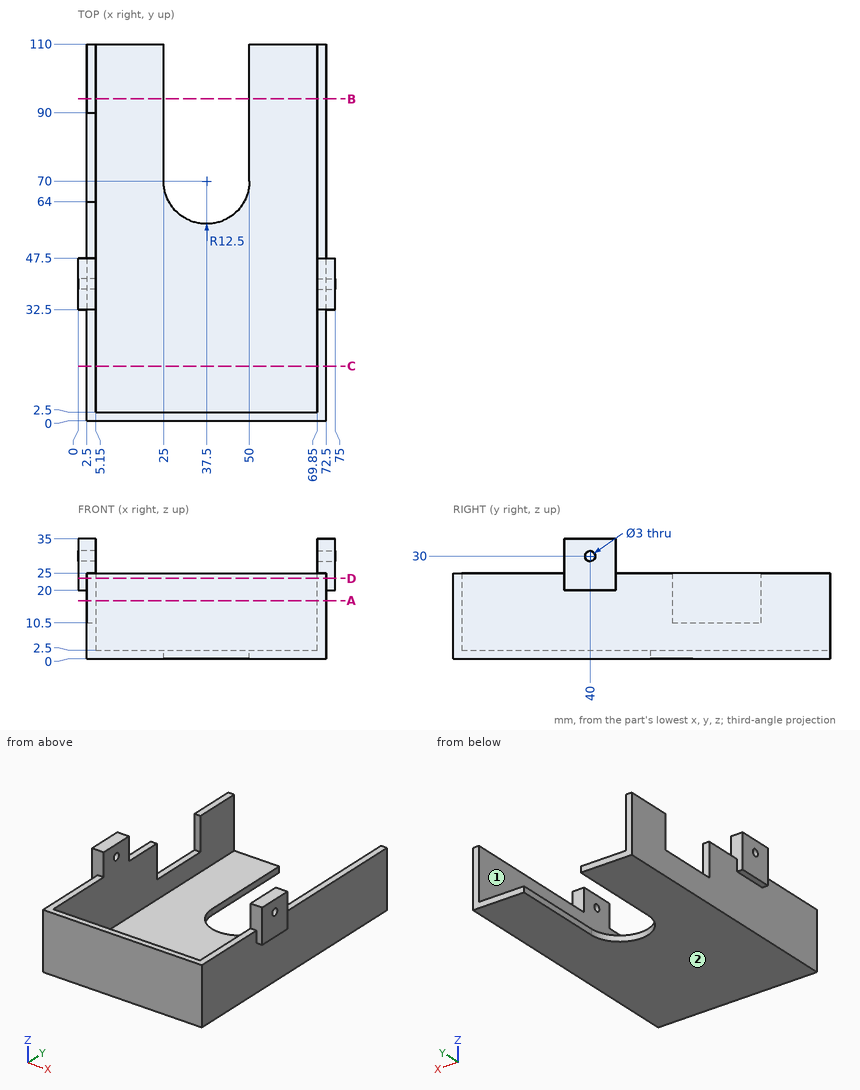
Geometry check sheet. Reference: drawing and pictorial views, mm from the part's lowest x, y, z. A direction names the side the tool comes from. Round coordinates to 2 decimals unless told otherwise and drop trailing zeros. Order: outer loops, then holes, each group sorted by start corner. A loop starts at its lowest first (then second) coordinate and runs counter-clockwise, first axis right, second up. Notation, with made-up numbers: (-26, -10) - (8, -10) arc R35 cw to (8, 23) - close; hole circle Ø10 at (26, 48.5). An arc over 180 degrees is marked (long way). Use a Markdown table: item, result. Add a question column.
1) Gauge pin test, flat ends, axial feed: P1, Ø1.3, axis at x = 3.5, y = 102, coming from the +Z side; P2, Ø0.8, axis at x = 4.5, y = 76.5, coming from the +Z side; P3, Ø5, axis at y = 40, z = 30, coming from the -X side; P4, Ø11, axis at x = 48, z = 14, coming from the +Y side. Record the tip position at first contact, or that the pin passes through.
2) Section check B-B (y = 94). Record the cut outline in (x, z).
3) Thickness scan on line 1 along X through (y, z) = (90, 7); line 2 along Y through (x, z) = (71.3, 30); line 3 along Z through (x, y) = (2.25, 40). Record the ranges inside material, lowest first.
4) Set-up check for the marked faces 1 and 2: record each of +Z, -Z, +X, -X, +Y, -Y from which the full face is reachable in a straight line by a thin tool's end or side.
5) Section check D-D (z = 23.5). Record the cut outline in (x, y).
6) Section check A-A (z = 17). Record the cut outline in (x, y), then the cut area to 3 significant figures.
7) Section check C-C (y = 16). Record the cut outline in (x, z).
Established:
| question | item | result |
|---|---|---|
| 1 | P1 | z = 25 |
| 1 | P2 | z = 10.5 |
| 1 | P3 | x = 0 |
| 1 | P4 | y = 2.5 |
| 2 | outline | (2.5, 0) - (25, 0) - (25, 2.5) - (5.15, 2.5) - (5.15, 25) - (2.5, 25) - close; (50, 0) - (72.5, 0) - (72.5, 25) - (69.85, 25) - (69.85, 2.5) - (50, 2.5) - close |
| 3 | line 1 | 2.5 to 5.15, 69.85 to 72.5 |
| 3 | line 2 | 32.5 to 38.5, 41.5 to 47.5 |
| 3 | line 3 | 20 to 28.5, 31.5 to 35 |
| 4 | face 1 | +Z, +Y |
| 4 | face 2 | -Z, +X, -X, +Y, -Y |
| 5 | outline | (0, 32.5) - (2.5, 32.5) - (2.5, 0) - (72.5, 0) - (72.5, 32.5) - (75, 32.5) - (75, 47.5) - (72.5, 47.5) - (72.5, 110) - (69.85, 110) - (69.85, 2.5) - (5.15, 2.5) - (5.15, 64) - (2.5, 64) - (2.5, 47.5) - (0, 47.5) - close; (2.5, 90) - (5.15, 90) - (5.15, 110) - (2.5, 110) - close |
| 6 | outline | (2.5, 0) - (72.5, 0) - (72.5, 110) - (69.85, 110) - (69.85, 2.5) - (5.15, 2.5) - (5.15, 64) - (2.5, 64) - close; (2.5, 90) - (5.15, 90) - (5.15, 110) - (2.5, 110) - close |
| 6 | area | 676 mm2 |
| 7 | outline | (2.5, 0) - (72.5, 0) - (72.5, 25) - (69.85, 25) - (69.85, 2.5) - (5.15, 2.5) - (5.15, 25) - (2.5, 25) - close |
